from build123d import *

# Parameters (mm, degrees)
SKETCH_1_R          = 1.5
EXTRUDE_1_DEPTH     = 3
SKETCH_3_R          = 9
SKETCH_3_R_2        = 8
EXTRUDE_2_DEPTH     = 18
SKETCH_4_W          = 18
SKETCH_4_H          = 2.480736202
CUT_EXTRUDE_1_DEPTH = 30


with BuildPart() as part:
    # 草图1 → 凸台-拉伸1 (new body)
    with BuildSketch(Plane(origin=(0, 0, 0), x_dir=(1, 0, 0), z_dir=(0, 1, 0))):
        with BuildLine():
            Line((-16.5, 15), (16.5, 15))
            Line((16.5, 15), (16.5, 9))
            ThreePointArc((16.5, 9), (11.982501162, 6.959373548), (9, 3))
            Line((9, 3), (9, -3))
            ThreePointArc((9, -3), (11.982501162, -6.959373548), (16.5, -9))
            Line((16.5, -9), (16.5, -15))
            Line((16.5, -15), (-16.5, -15))
            Line((-16.5, -15), (-16.5, -9))
            ThreePointArc((-16.5, -9), (-11.982501162, -6.959373548), (-9, -3))
            Line((-9, -3), (-9, 3))
            ThreePointArc((-9, 3), (-11.982501162, 6.959373548), (-16.5, 9))
            Line((-16.5, 9), (-16.5, 15))
        make_face()
        with Locations(Location((-13.5, 12.5, 0), (0, 0, 270))):
            Circle(SKETCH_1_R, mode=Mode.SUBTRACT)
        with Locations(Location((13.5, 12.5, 0), (0, 0, 270))):
            Circle(SKETCH_1_R, mode=Mode.SUBTRACT)
        with Locations(Location((13.5, -12.5, 0), (0, 0, 270))):
            Circle(SKETCH_1_R, mode=Mode.SUBTRACT)
        with Locations(Location((-13.5, -12.5, 0), (0, 0, 270))):
            Circle(SKETCH_1_R, mode=Mode.SUBTRACT)
    extrude(amount=EXTRUDE_1_DEPTH)

    # 草图3 → 凸台-拉伸2 (add)
    with BuildSketch(Plane(origin=(0, 2.772072144, 0.794878896), x_dir=(1, 0, 0), z_dir=(0, 0.9612616959383188, 0.27563735581699983))):
        with Locations(Location((0, 0.826912067, 0), (0, 0, 270))):
            Circle(SKETCH_3_R)
        with Locations(Location((0, 0.826912067, 0), (0, 0, 270))):
            Circle(SKETCH_3_R_2, mode=Mode.SUBTRACT)
    extrude(amount=-EXTRUDE_2_DEPTH)

    # 草图4 → 切除-拉伸1 (cut)
    with BuildSketch(Plane.XY.offset(15)):
        with Locations((0, 4.240368101)):
            Rectangle(SKETCH_4_W, SKETCH_4_H)
    extrude(amount=-CUT_EXTRUDE_1_DEPTH, mode=Mode.SUBTRACT)


solid = part.part
Source: CAD feature listing. Evaluate the final solid. Frame: model axes, mm. A direction names the side the tool comes from. Give positions to 0.01 mm unless a question says otherwise; leave off trailing zeros. Loops run counter-clockwise (first coordinate to the right, second up) from the corner with the lowest first, then second, coordinate; pieces in that order, holes last. Notation, with made-up numbers: (28.5, 25) -> (48.5, 25) arc R28 ccw to (48.5, 43) -> close; hole circle Ø4 at (84.5, -13). An arc over 180 degrees is marked (long way). Use a Markdown table: item, result. Add a question column.
1) Section query C-C, the plane x = -13.5. Return the cut outline in (y, z).
2) Section query D-D, the plane x = 7. Return the cut outline in (y, z).
3) Reachability of faces 4 (the face through (2.4, -9.87, 4.25)), 5 (the face through (-12.037, 1.479, 7.003)), 6 (the face through (0, 0, -11)), 7 (the face through (12.037, 1.479, -7.003)) from +Z, -Z, +X, -X, +Y, -Y: full face, straight path, thin tool, end or side. Return the list, or none.
4) First-contact query: pin 1 (1 mm diameter, centred on y = -4.5, z = -1, fed in from +X); pin 2 (10 mm diameter, centred on y = -8.5, z = 8.5, fed in from -X); pin 3 (8 mm diameter, centred on x = -10, z = -6, fed in from -Y). Flat tips, straight axial feed; report the tip coordinate or a pass-through.
5) Pull-direction query (Y, two-part tool) for faces 1 (the face through (0, 3, 0)), 2 (the face through (-16.5, 1, -12)), 3 (the face through (0, 0, -1)); classes: +Y half, -Y half, draft (parallel to the pull), parting line (faces both ways), or undercut.
6) Section query A-A, the plane z = 12.5. Return the cut outline in (x, y), then the cut area to 3 significant figures.
7) Line query: line 1 along X through (y, z) = (2.2, -12.5); line 2 along Y through (x, z) = (-4.5, -0.25); line 3 along X through (y, z) = (-8.5, -10). Output: solid intervals per line, ascending. Write a range as [from, to].
8) Section query B-B, the plane y = 0.75. Return the cut outline in (x, z), then the cut area to 3 significant figures.
Numbers:
| question | item | result |
|---|---|---|
| 1 | outline | (0, -15) -> (3, -15) -> (3, -14) -> (0, -14) -> close; (0, -11) -> (3, -11) -> (3, -7.96) -> (0, -7.96) -> close; (0, 7.96) -> (3, 7.96) -> (3, 11) -> (0, 11) -> close; (0, 14) -> (3, 14) -> (3, 15) -> (0, 15) -> close |
| 2 | outline | (-15.86, 0.48) -> (-15.37, -1.24) -> (0, 3.17) -> (0, -4.89) -> (-13.24, -8.68) -> (-12.74, -10.4) -> (0, -6.75) -> (0, -15) -> (3, -15) -> (3, 15) -> (0, 15) -> (0, 5.02) -> close |
| 3 | face 4 | none |
| 3 | face 5 | -X, +Y, -Y |
| 3 | face 6 | -Z |
| 3 | face 7 | +X, +Y, -Y |
| 4 | pin 1 | stops at x = 8.98 |
| 4 | pin 2 | stops at x = -6.39 |
| 4 | pin 3 | stops at y = -15.07 |
| 5 | face 1 | +Y half |
| 5 | face 2 | draft |
| 5 | face 3 | undercut |
| 6 | outline | (-16.5, 0) -> (-15, 0) -> (-15, 3) -> (-16.5, 3) -> close; (-12, 0) -> (12, 0) -> (12, 3) -> (-12, 3) -> close; (15, 0) -> (16.5, 0) -> (16.5, 3) -> (15, 3) -> close |
| 6 | area | 81.0 mm2 |
| 7 | line 1 | x = [-16.5, -15], [-12, 12], [15, 16.5] |
| 7 | line 2 | y = [0, 3] |
| 7 | line 3 | x = [-6.28, -4.74], [4.74, 6.28] |
| 8 | outline | (-16.5, -15) -> (16.5, -15) -> (16.5, -9) arc R10 cw to (9, -3) -> (9, 3) arc R10 cw to (16.5, 9) -> (16.5, 15) -> (-16.5, 15) -> (-16.5, 9) arc R10 cw to (-9, 3) -> (-9, -3) arc R10 cw to (-16.5, -9) -> close; hole circle Ø3 at (-13.5, -12.5); hole circle Ø3 at (-13.5, 12.5); hole circle Ø3 at (13.5, -12.5); hole circle Ø3 at (13.5, 12.5) |
| 8 | area | 750 mm2 |
